```python
from build123d import *

# Parameters (mm, degrees)
F0_R     = 9.525
F1_DEPTH = 6.35
F2_SIZE  = 2.54


with BuildPart() as f1:
    # F0 (on Top) → F1 (new body)
    with BuildSketch(Plane.XY):
        Polygon((50.8, 114.3), (-50.8, 114.3), (-50.8, 0), (-50.8, -114.3), (50.8, -114.3), (50.8, 0), align=None)
        with Locations((-25.4, 12.7)):
            Circle(F0_R, mode=Mode.SUBTRACT)
        with Locations((-25.4, 88.9)):
            Circle(F0_R, mode=Mode.SUBTRACT)
        with Locations((25.4, 12.7)):
            Circle(F0_R, mode=Mode.SUBTRACT)
        with Locations((25.4, 88.9)):
            Circle(F0_R, mode=Mode.SUBTRACT)
    extrude(amount=F1_DEPTH)

    # F2
    f2_edges = [f1.edges().sort_by_distance(p)[0] for p in [
        (-34.925, 88.9, 6.35),
        (15.875, 88.9, 6.35),
        (15.875, 12.7, 6.35),
        (-34.925, 12.7, 6.35),
    ]]
    chamfer(f2_edges, length=F2_SIZE)


solid = f1.part
```
Check sheet for the modelled part. Datum: model origin and axes. Units: mm. Coordinates: 2 decimals unless noted, no trailing zeros. Write each loop counter-clockwise with the first axis right and the second up, starting at its lowest first coordinate (ties: lowest second). Pieces come first, ordered by that corner, then holes. Notation, with made-up numbers: (-9, -4.5) - (4, -4.5) arc R35 ccw to (4, 27.5) - close; hole circle Ø11 at (22.5, 54). An arc over 180 degrees is marked (long way). One line per question, with ' | ' between items.
Item 1: Sectioned sample at C-C on z = 1.75. Record the boundary of the cut face in (x, y) (3 decimals).
Determined:
outline: (-50.8, -114.3) - (50.8, -114.3) - (50.8, 114.3) - (-50.8, 114.3) - close; hole circle Ø19.05 at (-25.4, 12.7); hole circle Ø19.05 at (-25.4, 88.9); hole circle Ø19.05 at (25.4, 12.7); hole circle Ø19.05 at (25.4, 88.9)
Item 2: Sectioned sample at A-A on x = -25.4. Record the boundary of the cut face in (y, z) (3 decimals).
Determined:
outline: (-114.3, 0) - (3.175, 0) - (3.175, 3.81) - (0.635, 6.35) - (-114.3, 6.35) - close; (22.225, 0) - (79.375, 0) - (79.375, 3.81) - (76.835, 6.35) - (24.765, 6.35) - (22.225, 3.81) - close; (98.425, 0) - (114.3, 0) - (114.3, 6.35) - (100.965, 6.35) - (98.425, 3.81) - close
Item 3: Mould release check, pull along Y, two halves, no side actions. Record for faces 1 (the face through (15.884, 13.119, 1.878)), 2 (the face through (1, 114.3, 3)), 3 (the face through (-50.8, 2, 3)): pulls with the +Y half, pulls with the -Y half, needs draft (parallel to the pull), parting line crosses it, or undercut.
Determined:
face 1: undercut | face 2: pulls with the +Y half | face 3: needs draft
Item 4: Sectioned sample at B-B on y = 88.9. Record the boundary of the cut face in (x, z) (3 decimals).
Determined:
outline: (-50.8, 0) - (-34.925, 0) - (-34.925, 3.81) - (-37.465, 6.35) - (-50.8, 6.35) - close; (-15.875, 0) - (15.875, 0) - (15.875, 3.81) - (13.335, 6.35) - (-13.335, 6.35) - (-15.875, 3.81) - close; (34.925, 0) - (50.8, 0) - (50.8, 6.35) - (37.465, 6.35) - (34.925, 3.81) - close
Item 5: Thickness scan on line 1 (Y direction, x = 25.4, z = 0.85) (3 decimals); line 2 (Y direction, x = 27, z = 2); line 3 (X direction, y = 19.5, z = 1). Record the ranges inside material, lowest first. Write a range as [from, to].
Determined:
line 1: y = [-114.3, 3.175], [22.225, 79.375], [98.425, 114.3] | line 2: y = [-114.3, 3.31], [22.09, 79.51], [98.29, 114.3] | line 3: x = [-50.8, -32.07], [-18.73, 18.73], [32.07, 50.8]
Item 6: Gauge pin test, flat ends, axial feed: P1, Ø6, axis at x = 37, y = -2.5, coming from the -Z side; P2, Ø4, axis at x = 21, y = 6, coming from the +Z side; P3, Ø22, axis at x = -25.4, y = 88.9, coming from the +Z side (3 decimals). Record the tip position at first contact, or that the pin passes through.
Determined:
P1: stops at z = 0 | P2: stops at z = 4.3 | P3: stops at z = 5.285
